Could you check a few things on this model? Use its own coordinates, in mm. Round coordinates to 2 decimals unless told otherwise and drop trailing zeros. Write each loop counter-clockwise with the first axis right and the second up, starting at its lowest first coordinate (ties: lowest second). Pieces come first, ordered by that corner, then holes. Notation, with made-up numbers: (-29, 48.25) -> (-17, 48.25) arc R15 cw to (-17, 67.25) -> close; hole circle Ø3 at (70.5, 58.25). An arc over 180 degrees is marked (long way). Return JSON: item names as keys, results as strings.
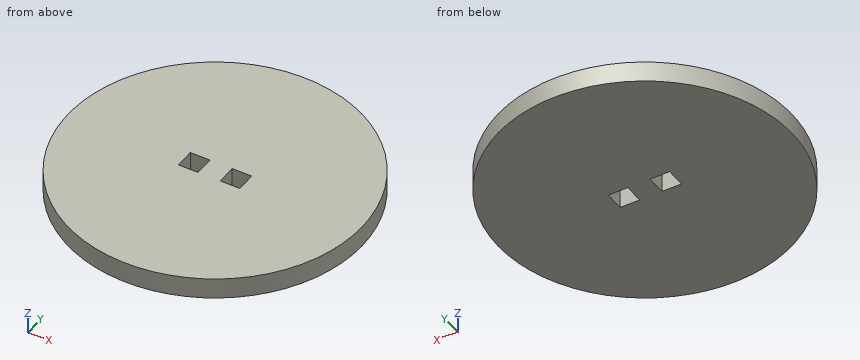
from build123d import *

# Parameters (mm, degrees)
SKETCH1_R           = 22.3266
SKETCH1_W           = 2.9718
SKETCH1_H           = 2.9718
BOSS_EXTRUDE1_DEPTH = 3.175


with BuildPart() as part:
    # Sketch1 → Boss-Extrude1 (new body)
    with BuildSketch(Plane.XY):
        Circle(SKETCH1_R)
        with Locations((-3.175, 0)):
            Rectangle(SKETCH1_W, SKETCH1_H, mode=Mode.SUBTRACT)
        with Locations((3.175, 0)):
            Rectangle(SKETCH1_W, SKETCH1_H, mode=Mode.SUBTRACT)
    extrude(amount=BOSS_EXTRUDE1_DEPTH)


solid = part.part
1) Will these pins go through, and if not, where does the flat tip stop? pin 1 Ø1.5 at (y, z) = (5, 1) entering from -X; pin 2 Ø1 at (y, z) = (17.5, 1) entering from -X.
Return value:
{"pin 1": "x = -21.92", "pin 2": "x = -14.47"}
2) I want a section at B-B, the plane x = 2.5. Please give me the cut outline in (y, z) (3 decimals).
Return value:
{"outline": "(-22.186, 0) -> (-1.486, 0) -> (-1.486, 3.175) -> (-22.186, 3.175) -> close; (1.486, 0) -> (22.186, 0) -> (22.186, 3.175) -> (1.486, 3.175) -> close"}
3) I want a section at A-A, the plane z = 1.55. Please give me the cut outline in (x, y).
Return value:
{"outline": "circle Ø44.65 at (0, 0); hole (-4.66, -1.49) -> (-1.69, -1.49) -> (-1.69, 1.49) -> (-4.66, 1.49) -> close; hole (1.69, -1.49) -> (4.66, -1.49) -> (4.66, 1.49) -> (1.69, 1.49) -> close"}
4) I want a section at D-D, the plane x = 8. Please give me the cut outline in (y, z) (3 decimals).
Return value:
{"outline": "(-20.844, 0) -> (20.844, 0) -> (20.844, 3.175) -> (-20.844, 3.175) -> close"}
5) I want a section at C-C, the plane y = -19. Please give me the cut outline in (x, z) (3 decimals), and give its area (3 significant figures).
Return value:
{"outline": "(-11.725, 0) -> (11.725, 0) -> (11.725, 3.175) -> (-11.725, 3.175) -> close", "area": "74.5 mm²"}
6) If I drill on probe 1 along X at (y, z) = (-0.5, 0.3); probe 2 along Y at (x, z) = (0, 2.45); probe 3 along X at (y, z) = (7, 2.3), over which ranges is the centre line in solid material (lowest first)? Write a range as [from, to].
Return value:
{"probe 1": "[-22.32, -4.66], [-1.69, 1.69], [4.66, 22.32]", "probe 2": "[-22.33, 22.33]", "probe 3": "[-21.2, 21.2]"}
